The listing builds one solid part. Answer for the finished solid, in the listing's coordinates (mm). A direction names the side the tool comes from. Give positions to 0.01 mm unless a question says otherwise; leave off trailing zeros. Order: outer loops, then holes, each group sorted by start corner. A loop starts at its lowest first (then second) coordinate and runs counter-clockwise, first axis right, second up. Notation, with made-up numbers: M 20,55.5 L 51,55.5 A24 ccw 51,79.5 Z; hole C -36.75,66.25 d4. An arc over 180 degrees is marked long. Answer as a JSON object with one key per item and string values. Group by question number.
Autodesk Inventor part; units mm, degrees
ref_plane "YZ Plane" through (0, 0, 0) normal (1, 0, 0) x (0, 1, 0)
ref_plane "XZ Plane" through (0, 0, 0) normal (0, 1, 0) x (-1, 0, 0)
ref_plane "XY Plane" through (0, 0, 0) normal (0, 0, 1) x (1, 0, 0)
sketch "Sketch1" plane through (0, 0, 0) normal (0, 1, 0) x (-1, 0, 0)
  line L0 (0, 0) -> (0, -50.8)
  line L1 (0, -50.8) -> (-50.8, -50.8)
  line L2 (-50.8, -50.8) -> (-50.8, -44.45)
  line L3 (-50.8, -44.45) -> (-6.35, -44.45)
  line L4 (-6.35, -44.45) -> (-6.35, 0)
  line L5 (-6.35, 0) -> (0, 0)
  dimension "d0" = 6.35
  dimension "d1" = 50.8
extrude "Extrusion1" add sketch "Sketch1" along normal blind 152.4
sketch "Sketch4" plane through (6.35, 0, -44.45) normal (0, 0, 1) x (1, 0, 0)
  line L0 (44.45, 0) -> (0, 0)
  line L1 (0, 0) -> (0, 152.4)
  line L2 (44.45, 0) -> (0, 0)
  line L3 (0, 0) -> (0, 44.45)
  line L4 (0, 44.45) -> (44.45, 44.45)
  line L5 (44.45, 44.45) -> (44.45, 0)
  point P0 (-6.35, 0)
  dimension "d8" = 44.45
extrude "Extrusion3" cut sketch "Sketch4" against normal through all
sketch "Sketch5" plane through (6.35, 152.4, -44.45) normal (0, 0, 1) x (1, 0, 0)
  line L0 (44.45, -107.95) -> (44.45, 0)
  line L1 (44.45, 0) -> (-6.35, 0)
  line L2 (44.45, -107.95) -> (19.05, -107.95)
  line L3 (19.05, -107.95) -> (19.05, 0)
  line L4 (19.05, 0) -> (44.45, 0)
  line L5 (44.45, 0) -> (44.45, -107.95)
  point P0 (-6.35, -152.4)
  dimension "d11" = 25.4
extrude "Extrusion4" cut sketch "Sketch5" against normal through all
sketch "Sketch6" plane through (0, 0, -50.8) normal (-1, 0, 0) x (0, 0, 1)
  line L0 (0, 152.4) -> (50.8, 152.4)
  line L1 (0, 0) -> (0, 152.4)
  line L2 (50.8, 0) -> (50.8, 152.4)
  point P0 (28.575, 127)
  dimension "d14" = 25.4
  dimension "d23" = 22.225
hole "Hole1" at (0, 127, -22.225) direction (1, 0, 0) diameter 10.0838 end through all
properties part number "LiftAngleBracketExtensionRight" material "Aluminum 6061"
Item 1: A tool of negligible diameter and unlimited length cuts with its end or side. For faces 5 (the flat face through (16, 98, -44.45)), 6 (the flat face through (16, 44.45, -48)), 7 (the flat face through (0, 75, -25)), from which of +Z, -Z, +X, -X, +Y, -Y can it reach the whole face along a straight path? Write none if from no direction.
Item 2: Determine the mould class of faces 1 (the cylindrical face through (3.219, 126.778, -27.262)), 2 (the flat face through (6.35, 75, -26)), 3 (the flat face through (3, 0, -25)), 4 (the flat face through (5, 152.4, -31)) for opening direction Y: released by +Y, released by -Y, zero draft, split by the parting line, or undercut.
Item 3: Section A-A (y = 127) is taken. Determine the outline of the cut face in (x, z), and give its area (3 significant figures).
Item 4: Section B-B (z = -46.5) is taken. Determine the outline of the cut face in (x, y), and give its area (3 significant figures).
Item 5: Section C-C (y = 21) is taken. Determine the outline of the cut face in (x, z).
Item 6: Section D-D (x = 9) is taken. Determine the outline of the cut face in (y, z).
Item 7: Flat-ended cylindrical pins translate along their axes: P1, Ø1.9, axis at x = 15.5, z = -48, coming from the -Y side; P2, Ø9.5, axis at x = 12, y = 114, coming from the +Z side; P3, Ø1, axis at y = 23.5, z = -19, coming from the +X side. Find the tip coordinate at first contact, or state that the pin passes through.
Item 8: Consider probe 1 along Z at (x, y) = (2.5, 127); probe 2 along X at (y, z) = (133, -13); probe 3 along Y at (x, z) = (8, -46). Determine where each line is inside the solid, lowest interval first. Write a range as from..to.
Values found:
{
 "1": {"face 5": "+Z, +X, +Y, -Y", "face 6": "+Z, -Z, +X, -Y", "face 7": "+Z, -Z, -X, +Y, -Y"},
 "2": {"face 1": "undercut", "face 2": "zero draft", "face 3": "released by -Y", "face 4": "released by +Y"},
 "3": {"outline": "M 0,-50.8 L 25.4,-50.8 L 25.4,-44.45 L 6.35,-44.45 L 6.35,-27.27 L 0,-27.27 Z; M 0,-17.18 L 6.35,-17.18 L 6.35,0 L 0,0 Z", "area": "380 mm^2"},
 "4": {"outline": "M 0,0 L 6.35,0 L 6.35,44.45 L 25.4,44.45 L 25.4,152.4 L 0,152.4 Z", "area": "3,020 mm^2"},
 "5": {"outline": "M 0,-50.8 L 6.35,-50.8 L 6.35,0 L 0,0 Z"},
 "6": {"outline": "M 44.45,-50.8 L 152.4,-50.8 L 152.4,-44.45 L 44.45,-44.45 Z"},
 "7": {"P1": "stops at y = 44.45", "P2": "stops at z = -44.45", "P3": "stops at x = 6.35"},
 "8": {"probe 1": "z = -50.8..-27.27, -17.18..0", "probe 2": "x = 0..6.35", "probe 3": "y = 44.45..152.4"}
}
